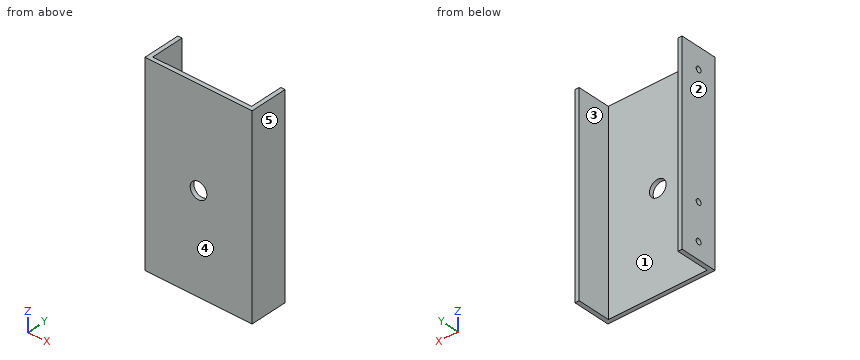
```python
from build123d import *

# Parameters (mm, degrees)
BOSS_EXTRUDE1_DEPTH = 35
SKETCH2_R           = 3
CUT_EXTRUDE1_DEPTH  = 43.186964811
CUT_EXTRUDE3_REACH  = 55.826
SKETCH4_R           = 1


with BuildPart() as part:
    # Sketch1 → Boss-Extrude1 (new, symmetric)
    with BuildSketch(Plane.XY):
        Polygon((-19.3, 13.5), (-19.3, 0), (19.3, 0), (19.3, 13.5), (17.8, 13.5), (17.8, 1.5), (-17.8, 1.5), (-17.8, 13.5), align=None)
    extrude(amount=BOSS_EXTRUDE1_DEPTH, both=True)

    # Sketch2 → Cut-Extrude1 (cut, through all)
    with BuildSketch(Plane.XZ):
        with Locations(Location((0, 0, 0), (0, 0, 270))):
            Circle(SKETCH2_R)
    extrude(amount=-CUT_EXTRUDE1_DEPTH, mode=Mode.SUBTRACT)

    # Sketch4 → Cut-Extrude3 (cut, up to next)
    with BuildSketch(Plane.ZY.offset(19.3), mode=Mode.PRIVATE) as cut_extrude3_sk1:
        with Locations(Location((-29, 6.75, 0), (0, 0, 270))):
            Circle(SKETCH4_R)
    cut_extrude3_tool1 = extrude(cut_extrude3_sk1.sketch, amount=-CUT_EXTRUDE3_REACH, mode=Mode.PRIVATE) & part.part
    # Sketch4 → Cut-Extrude3 (cut, up to next)
    with BuildSketch(Plane.ZY.offset(19.3), mode=Mode.PRIVATE) as cut_extrude3_sk2:
        with Locations(Location((-16, 6.75, 0), (0, 0, 270))):
            Circle(SKETCH4_R)
    cut_extrude3_tool2 = extrude(cut_extrude3_sk2.sketch, amount=-CUT_EXTRUDE3_REACH, mode=Mode.PRIVATE) & part.part
    # Sketch4 → Cut-Extrude3 (cut, up to next)
    with BuildSketch(Plane.ZY.offset(19.3), mode=Mode.PRIVATE) as cut_extrude3_sk3:
        with Locations(Location((27.5, 6.75, 0), (0, 0, 270))):
            Circle(SKETCH4_R)
    cut_extrude3_tool3 = extrude(cut_extrude3_sk3.sketch, amount=-CUT_EXTRUDE3_REACH, mode=Mode.PRIVATE) & part.part
    add(cut_extrude3_tool1.solids().sort_by_distance((-19.3, 6.75, -29))[0], mode=Mode.SUBTRACT)
    add(cut_extrude3_tool2.solids().sort_by_distance((-19.3, 6.75, -16))[0], mode=Mode.SUBTRACT)
    add(cut_extrude3_tool3.solids().sort_by_distance((-19.3, 6.75, 27.5))[0], mode=Mode.SUBTRACT)


solid = part.part
```
CAD build for the part. Positions are in the model's coordinates, mm. Face numbers are marked on the shaded views. A direction names the side the tool comes from. Coordinates: 2 decimals unless noted, no trailing zeros. Order: outer loops, then holes, each group sorted by start corner. A loop starts at its lowest first (then second) coordinate and runs counter-clockwise, first axis right, second up. Notation, with made-up numbers: (1.5, 71) - (27.5, 71) arc R18 ccw to (27.5, 101) - close; hole circle Ø4 at (21.5, 54.25). An arc over 180 degrees is marked (long way). Use a Markdown table: item, result. Add a question column.
(1) Drill centre lines: line 1 along Z through (x, y) = (-18.4, 6.75); line 2 along X through (y, z) = (6.75, 3); line 3 along X through (y, z) = (1, 0). Where is each one in solid material? Low to high. Write a range as [from, to].
(2) Pull direction X, two halves, no side cores. Call the marked faces 3, 4 and 5: +X half, -X half, draft (parallel to the pull), parting line (faces both ways), or undercut.
(3) Flat gauge pins, fed straight in: pin 1 (5 mm diameter, centred on x = -1.5, z = 17, fed in from +Y); pin 2 (1.2 mm diameter, centred on y = 6.75, z = -29, fed in from -X). Where does each tip first touch, or does it go through?
(4) Which spindle directions (+Z, -Z, +X, -X, +Y, -Y) get a long thin tool onto all of the face, cutting with end or side? Do the marked faces 1 and 2. Say none if no direction does.
(5) Saw through at B-B (y = 3.25). Give the cut face in (x, z), then the cut area to 3 significant figures.
(6) Saw through at D-D (z = 0). Give the cut face in (x, y).
(7) Saw through at A-A (x = 0). Give the cut face in (y, z), then the cut area to 3 significant figures.
(8) Saw through at C-C (z = -16). Give the cut face in (x, y).
Solved:
| question | item | result |
|---|---|---|
| 1 | line 1 | z = [-35, -30], [-28, -17], [-15, 26.5], [28.5, 35] |
| 1 | line 2 | x = [-19.3, -17.8], [17.8, 19.3] |
| 1 | line 3 | x = [-19.3, -3], [3, 19.3] |
| 2 | face 3 | undercut |
| 2 | face 4 | draft |
| 2 | face 5 | +X half |
| 3 | pin 1 | stops at y = 1.5 |
| 3 | pin 2 | stops at x = 17.8 |
| 4 | face 1 | +Z, -Z, +Y |
| 4 | face 2 | +Z, -Z, -X, +Y, -Y |
| 5 | outline | (-19.3, -35) - (-17.8, -35) - (-17.8, 35) - (-19.3, 35) - close; (17.8, -35) - (19.3, -35) - (19.3, 35) - (17.8, 35) - close |
| 5 | area | 210 mm² |
| 6 | outline | (-19.3, 0) - (-3, 0) - (-3, 1.5) - (-17.8, 1.5) - (-17.8, 13.5) - (-19.3, 13.5) - close; (3, 0) - (19.3, 0) - (19.3, 13.5) - (17.8, 13.5) - (17.8, 1.5) - (3, 1.5) - close |
| 7 | outline | (0, -35) - (1.5, -35) - (1.5, -3) - (0, -3) - close; (0, 3) - (1.5, 3) - (1.5, 35) - (0, 35) - close |
| 7 | area | 96.0 mm² |
| 8 | outline | (-19.3, 0) - (19.3, 0) - (19.3, 13.5) - (17.8, 13.5) - (17.8, 1.5) - (-17.8, 1.5) - (-17.8, 5.75) - (-19.3, 5.75) - close; (-19.3, 7.75) - (-17.8, 7.75) - (-17.8, 13.5) - (-19.3, 13.5) - close |
